Read the model definition and answer for the solid it produces. Units are mm, in the model's axes. Face numbers are marked on the shaded views. A direction names the side the tool comes from. Coordinates: 2 decimals unless noted, no trailing zeros. Write each loop counter-clockwise with the first axis right and the second up, starting at its lowest first coordinate (ties: lowest second). Pieces come first, ordered by that corner, then holes. Notation, with made-up numbers: (-22.5, 64) -> (23.5, 64) arc R16 cw to (23.5, 85) -> close; hole circle Ø2 at (22.5, 11.5). An arc over 180 degrees is marked (long way). Answer as a JSON object with one key per item and string values. Group by question number.
(1) Flat-ended cylindrical pins translate along their axes: P1, Ø1.8, axis at x = -8.5, y = 3.5, coming from the -Z side; P2, Ø1.1, axis at x = -1, y = -3.5, coming from the +Z side; P3, Ø0.8, axis at y = 1.5, z = -15.5, coming from the -X side; P4, Ø1.1, axis at x = -15, y = -4, coming from the -Z side. Find the tip coordinate at first contact, or state that the pin passes through.
(2) Find section D-D (x = -13.25). Give the vertices of the cut face in (y, z).
(3) Find section B-B (y = -3.25). Give the vertices of the cut face in (x, z), then the cut area to 3 significant figures.
(4) Straight lines are drawn through the part: L1, parallel to Z at x = -8, y = -0.35; L2, parallel to Z at x = -8, y = 1; L3, parallel to X at y = -1.25, z = -14.75. For each, find the intervals that lie inside material, in ascending order.
(5) Which of the six approach directions +Z, -Z, +X, -X, +Y, -Y give full straight-line access (tool end or side, diameter ignored) to the marked faces 1, 2 and 3?
(6) For a pull along Z with two mould halves and no side action, classify the marked faces 4, 5 and 6 as +Z half, -Z half, draft (parallel to the pull), parting line (faces both ways), or undercut.
(7) Find section C-C (y = 1). Give the vertices of the cut face in (x, z).
(8) Find section A-A (y = -1.5). Give the vertices of the cut face in (x, z).
Autodesk Inventor part; units mm, degrees
ref_plane "YZ Plane" through (0, 0, 0) normal (1, 0, 0) x (0, 1, 0)
ref_plane "XZ Plane" through (0, 0, 0) normal (0, 1, 0) x (-1, 0, 0)
ref_plane "XY Plane" through (0, 0, 0) normal (0, 0, 1) x (1, 0, 0)
sketch "Sketch5" plane through (0, 0, 0) normal (0, 1, 0) x (-1, 0, 0)
  line L0 (-3.1299, 16.302) -> (-3.1299, -27.8812) construction
  line L1 (-3.1299, -27.8812) -> (-19.0358, -27.8812) construction
  line L2 (-19.0358, -27.8812) -> (-19.0358, 16.302) construction
  line L3 (-19.0358, 16.302) -> (-3.1299, 16.302) construction
  line L4 (0, 0) -> (16, 0)
  line L5 (8, 0) -> (8, -24.9508) construction
  line L6 (16, 0) -> (8, -13)
  line L7 (8, -13) -> (0, 0)
  circle A0 centre (8, -15) radius 2.1568
  line L8 (0, 0) -> (0, -12.5098) construction
  point P0 (7.9048, -12.8453)
  point P1 (8.0952, -12.8453)
  dimension "d36" = 16
  dimension "d42" = 13
  dimension "d43" = 2
extrude "Extrusion4" add sketch "Sketch5" along normal blind 5
sketch "Sketch6" plane through (0, 5, 0) normal (0, 1, 0) x (1, 0, 0)
  arc A0 (-7.9048, 12.8453) -> (-8.0952, 12.8453) centre (-8, 15) ccw
  circle A1 centre (-8, 15) radius 1.6568
  line L0 (-16, 0) -> (0, 0)
  line L1 (-16, 0) -> (0, 0) construction
  line L2 (-14.2104, 1) -> (-8, 11.092)
  line L3 (-8.0952, 12.8453) -> (-16, 0)
  line L4 (-8, 11.092) -> (-1.7896, 1)
  line L5 (0, 0) -> (-7.9048, 12.8453)
  line L6 (-14.2104, 1) -> (-1.7896, 1)
  line L7 (-8, 15) -> (-8, 0) construction
  dimension "d46" = 0.5
  dimension "d52" = 1
  dimension "d53" = 1
extrude "Extrusion5" [suppressed]
fillet "Fillet1" radius 1 2 edges at (0, 2.5, 0) (-16, 2.5, 0)
sketch "Sketch9" plane through (0, 0, 0) normal (0, -1, 0) x (1, 0, 0)
  line L0 (-15.5, 3) -> (-0.5, 3)
  line L1 (-0.5, 3) -> (-0.5, -19)
  line L2 (-0.5, -19) -> (-15.5, -19)
  line L3 (-15.5, -19) -> (-15.5, 3)
  line L4 (-15.5, 3) -> (-0.5, -19) construction
  line L5 (-0.5, 3) -> (-15.5, -19) construction
  line L6 (-14.2104, 0) -> (-1.7896, 0)
  line L7 (-8, -15) -> (-8, 0) construction
  arc A0 (-8.0952, -12.8453) -> (-7.9048, -12.8453) centre (-8, -15) ccw construction
  circle A1 centre (-8, -15) radius 2.1568 construction
  point P0 (0, 0)
  point P1 (-8, -8)
  dimension "d75" = 15
  dimension "d76" = 22
  dimension "d77" = 3
extrude "Extrusion7" add sketch "Sketch9" along normal blind 3
sketch "Sketch10" plane through (0, -3, 0) normal (0, -1, 0) x (1, 0, 0)
  line L0 (-0.5, -19) -> (-0.5, 3)
  line L1 (-0.5, -0.75) -> (-1.5, -0.75)
  line L2 (-1.5, -0.75) -> (-1.5, -3.75)
  line L3 (-1.5, -3.75) -> (-0.5, -3.75)
  line L4 (-0.5, -3.75) -> (-0.5, -0.75)
  line L5 (-15.5, 3) -> (-15.5, -19)
  line L6 (-15.5, -0.75) -> (-14.5, -0.75)
  line L7 (-14.5, -0.75) -> (-14.5, -3.75)
  line L8 (-14.5, -3.75) -> (-15.5, -3.75)
  line L9 (-15.5, -3.75) -> (-15.5, -0.75)
  line L10 (-0.5, 3) -> (-15.5, 3)
  point P0 (0, 0)
  point P1 (-15.5, -3.75)
  point P2 (-0.5, -3.75)
  dimension "d80" = 1
  dimension "d81" = 3
  dimension "d82" = 1
  dimension "d83" = 3
  dimension "d84" = 3.75
  dimension "d85" = 3.75
extrude "Extrusion8" add sketch "Sketch10" along normal blind 1.6
sketch "Sketch11" plane through (0, -3, 0) normal (0, -1, 0) x (1, 0, 0)
  line L0 (-9.25, -1.75) -> (-6.75, -1.75)
  line L1 (-6.75, -1.75) -> (-6.75, -3.25)
  line L2 (-6.75, -3.25) -> (-9.25, -3.25)
  line L3 (-9.25, -3.25) -> (-9.25, -1.75)
  line L4 (-8, 0) -> (-8, -15.1696) construction
  line L5 (-15.5, -19) -> (-0.5, -19) construction
  line L6 (-8, -19) -> (-8, 3) construction
  line L7 (-0.5, 3) -> (-15.5, 3) construction
  line L8 (-1.5, -0.75) -> (-1.5, -3.75)
  line L9 (-14.5, -3.75) -> (-14.5, -0.75)
  line L10 (-0.5, -0.75) -> (-1.5, -0.75)
  line L11 (-15.5, -3.75) -> (-15.5, -19)
  line L12 (-6.75, -14.75) -> (-9.25, -14.75)
  line L13 (-9.25, -14.75) -> (-9.25, -16.25)
  line L14 (-9.25, -16.25) -> (-6.75, -16.25)
  line L15 (-6.75, -16.25) -> (-6.75, -14.75)
  line L16 (-6.75, -14.75) -> (-9.25, -16.25) construction
  line L17 (-9.25, -14.75) -> (-6.75, -16.25) construction
  line L18 (-1.5, -3.75) -> (-0.5, -3.75)
  point P0 (0, 0)
  point P1 (-8, -1.75)
  point P2 (-9.25, -2.5)
  point P3 (-8, -3.25)
  point P4 (-8, 0)
  point P5 (-8, -8)
  point P6 (-6.75, -2.5)
  point P7 (-8, -15.5)
  point P8 (-6.75, -15.5)
  dimension "d129" = 7.5
  dimension "d133" = 1.5
  dimension "d136" = 2.5
  dimension "d137" = 1.5
  dimension "d138" = 13
  dimension "d141" = 0.5
extrude "Extrusion9" cut sketch "Sketch11" against normal blind 16
sketch "Sketch13" plane through (0, -3, 0) normal (0, -1, 0) x (1, 0, 0)
  line L0 (-1.5, 2) -> (-14.5, 2)
  line L1 (-14.5, 2) -> (-14.5, -18)
  line L2 (-14.5, -18) -> (-1.5, -18)
  line L3 (-1.5, -18) -> (-1.5, 2)
  line L4 (-0.5, 3) -> (-15.5, 3)
  line L5 (-0.5, -0.75) -> (-0.5, 3)
  line L6 (-15.5, 3) -> (-15.5, -0.75)
  line L7 (-15.5, -19) -> (-0.5, -19)
  point P0 (0, 0)
  point P1 (-15.5, 1.125)
  dimension "d106" = 1
  dimension "d107" = 1
  dimension "d108" = 1
  dimension "d109" = 1
extrude "Extrusion11" cut sketch "Sketch13" against normal blind 2
sketch "Sketch14" plane through (0, -1, 0) normal (0, -1, 0) x (1, 0, 0)
  line L0 (-9.25, -14.75) -> (-9.25, -16.25) construction
  line L1 (-9.25, -15.5) -> (-6.75, -15.5) construction
  line L2 (-6.75, -16.25) -> (-6.75, -14.75) construction
  line L3 (-9.25, -16.25) -> (-6.75, -16.25) construction
  line L4 (-8, -16.25) -> (-8, -1.75) construction
  line L5 (-6.75, -1.75) -> (-9.25, -1.75) construction
  line L6 (-9.25, -1.75) -> (-9.25, -3.25) construction
  line L7 (-9.25, -2.5) -> (-6.75, -2.5) construction
  line L8 (-6.25, -16.25) -> (-9.75, -16.25)
  line L9 (-9.75, -16.25) -> (-9.75, -14.75)
  line L10 (-9.75, -14.75) -> (-6.25, -14.75)
  line L11 (-6.25, -14.75) -> (-6.25, -16.25)
  line L12 (-6.25, -16.25) -> (-9.75, -14.75) construction
  line L13 (-9.75, -16.25) -> (-6.25, -14.75) construction
  line L14 (-6.25, -1.75) -> (-9.75, -1.75)
  line L15 (-9.75, -1.75) -> (-9.75, -3.25)
  line L16 (-9.75, -3.25) -> (-6.25, -3.25)
  line L17 (-6.25, -3.25) -> (-6.25, -1.75)
  line L18 (-6.25, -1.75) -> (-9.75, -3.25) construction
  line L19 (-9.75, -1.75) -> (-6.25, -3.25) construction
  point P0 (0, 0)
  point P1 (-8, -15.5)
  point P2 (-8, -2.5)
  dimension "d139" = 3.5
  dimension "d140" = 1.5
extrude "Extrusion12" cut sketch "Sketch14" against normal blind 1
sketch "Sketch15" plane through (0, -1, 0) normal (0, -1, 0) x (1, 0, 0)
  circle A0 centre (-8, -8.25) radius 1.25
  line L0 (-8, 0) -> (-8, -15) construction
  circle A1 centre (-8, -8.25) radius 1.95
  line L1 (-14.5, 2) -> (-1.5, 2)
  line L2 (-9.25, -3.25) -> (-6.75, -3.25)
  point P0 (0, 0)
  point P1 (-10.0959, -3.25)
  point P2 (-13.4041, -3.25)
  point P3 (-6.25, -3.25)
  point P4 (-9.75, -3.25)
  dimension "d117" = 2.5
  dimension "d118" = 0.7
  dimension "d131" = 10.25
extrude "Extrusion13" add sketch "Sketch15" along normal blind 2 contours A0 | A1
sketch "Sketch17" plane through (0, -1, 0) normal (0, -1, 0) x (1, 0, 0)
  point P0 (0, 0)
sketch "Sketch16" plane through (-8, -3, -8.25) normal (0, -1, 0) x (1, 0, 0)
  circle A0 centre (0, 0) radius 1.95
  circle A1 centre (0, 0) radius 1.25
  point P0 (8, 8.25)
  point P1 (-1.9339, 0.25)
  point P2 (1.9339, 0.25)
  dimension "d123" = 2.5
  dimension "d60" = 2.5
  dimension "d61" = 0.7
  dimension "d62" = 2.5
  dimension "d63" = 1.5
  dimension "d68" = 13
  dimension "d69" = 3.75
  dimension "d70" = 3.75
  dimension "d72" = 3.75
  dimension "d0" = 15
  dimension "d2" = 10
  dimension "d11" = 5
  dimension "d12" = 1.8
extrude "Extrusion14" cut sketch "Sketch16" against normal blind 5 contours A1
properties part number "NOTGATE2"
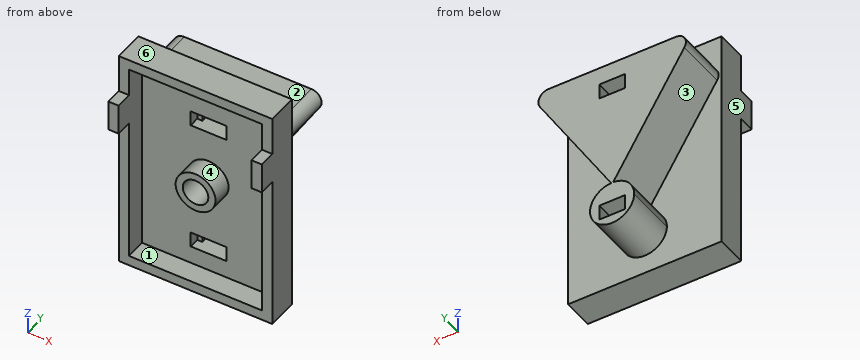
Results below:
{
 "1": {"P1": "stops at z = -17.16", "P2": "stops at z = 3", "P3": "stops at x = -10.15", "P4": "stops at z = -3.75"},
 "2": {"outline": "(-3, -19) -> (0, -19) -> (0, -4.47) -> (5, -4.47) -> (5, 0) -> (0, 0) -> (0, 3) -> (-3, 3) -> (-3, 2) -> (-1, 2) -> (-1, -18) -> (-3, -18) -> close"},
 "3": {"outline": "(-15.5, -3.75) -> (-14.5, -3.75) -> (-14.5, -0.75) -> (-15.5, -0.75) -> close; (-1.5, -3.75) -> (-0.5, -3.75) -> (-0.5, -0.75) -> (-1.5, -0.75) -> close", "area": "6.00 mm2"},
 "4": {"L1": "z = -19 to -16.25, -14.75 to -9.5, -7 to -3.25, -1.75 to 3", "L2": "z = -17.16 to -16.25, -14.75 to -9.5, -7 to -3.25, -1.75 to 0", "L3": "x = -15.5 to -14.5, -1.5 to -0.5"},
 "5": {"face 1": "-Y", "face 2": "+Z, +X, -X, +Y", "face 3": "-X, +Y"},
 "6": {"face 4": "undercut", "face 5": "draft", "face 6": "+Z half"},
 "7": {"outline": "(-15.06, -1.52) -> (-8.1, -12.85) arc R2.16 ccw (long way) to (-7.9, -12.85) -> (-0.94, -1.52) arc R1 ccw to (-1.79, 0) -> (-14.21, 0) arc R1 ccw to start; hole (-9.25, -16.25) -> (-6.75, -16.25) -> (-6.75, -14.75) -> (-9.25, -14.75) -> close; hole circle Ø2.5 at (-8, -8.25); hole (-9.25, -3.25) -> (-6.75, -3.25) -> (-6.75, -1.75) -> (-9.25, -1.75) -> close"},
 "8": {"outline": "(-15.5, -19) -> (-0.5, -19) -> (-0.5, 3) -> (-15.5, 3) -> close; circle Ø3.9 at (-8, -8.25); hole (-14.5, -18) -> (-1.5, -18) -> (-1.5, 2) -> (-14.5, 2) -> close; hole circle Ø2.5 at (-8, -8.25)"}
}
